from build123d import *

# Parameters (mm, degrees)
F1_DEPTH = 12.7
F2_DEPTH = 12.7
F4_DEPTH = 25.4
F6_DEPTH = 25.4
F8_DEPTH = 25.4


with BuildPart() as f1:
    # F0 (on Right) → F1 (new body)
    with BuildSketch(Plane.YZ):
        Polygon((304.799962, -64.221394), (304.799962, 304.800038), (266.7, 304.85419), (-42.510699, -10.741028), (-60.690689, -14.973944), (-60.690689, -19.789347), (-60.690689, -29.296394), (-60.690689, -64.221394), align=None)
        Polygon((-86.090689, -64.221394), (-60.690689, -64.221394), (-60.690689, -29.296394), (-60.690689, -19.789347), (-60.690689, -14.973944), (-86.090689, -14.973944), align=None)
    extrude(amount=F1_DEPTH)

    # F0 (on Right) → F2 (join)
    with BuildSketch(Plane.YZ):
        Polygon((304.799962, -64.221394), (304.799962, 304.800038), (266.7, 304.85419), (-42.510699, -10.741028), (-60.690689, -14.973944), (-60.690689, -19.789347), (-60.690689, -29.296394), (-60.690689, -64.221394), align=None)
        Polygon((-86.090689, -64.221394), (-60.690689, -64.221394), (-60.690689, -29.296394), (-60.690689, -19.789347), (-60.690689, -14.973944), (-86.090689, -14.973944), align=None)
    extrude(amount=F2_DEPTH)

    # F3 (on face) → F4 (cut)
    with BuildSketch(Plane.YZ.offset(12.7)):
        with BuildLine():
            Line((260.440068, 273.135901), (272.189458, 261.271445))
            ThreePointArc((272.189458, 261.271445), (279.866661, 265.037294), (282.611404, 273.135901))
            Line((282.611404, 273.135901), (282.614132, 279.79518))
            ThreePointArc((282.614132, 279.79518), (285.773725, 284.060884), (280.770869, 285.835901))
            Line((280.770869, 285.835901), (276.240647, 285.835901))
            ThreePointArc((276.240647, 285.835901), (276.167259, 285.912573), (276.174208, 286.018478))
            ThreePointArc((276.174208, 286.018478), (275.105821, 290.411047), (270.654796, 289.620796))
            Line((270.654796, 289.620796), (267.401841, 288.920168))
            ThreePointArc((267.401841, 288.920168), (266.952991, 289.962034), (266.735415, 291.075412))
            Line((266.735415, 291.075412), (266.735415, 304.926464))
            Line((266.735415, 304.926464), (243.648279, 281.326502))
            Line((243.648279, 281.326502), (252.004404, 281.326502))
            ThreePointArc((252.004404, 281.326502), (253.441245, 280.731343), (254.036404, 279.294502))
            Line((254.036404, 279.294502), (254.036404, 273.135901))
            Line((254.036404, 273.135901), (260.440068, 273.135901))
        make_face()
        with BuildLine():
            Line((177.841234, 200.373568), (177.841234, 214.224619))
            Line((177.841234, 214.224619), (154.754098, 190.624658))
            Line((154.754098, 190.624658), (163.110223, 190.624658))
            ThreePointArc((163.110223, 190.624658), (164.547063, 190.029499), (165.142223, 188.592658))
            Line((165.142223, 188.592658), (165.142223, 182.434057))
            Line((165.142223, 182.434057), (171.545887, 182.434057))
            Line((171.545887, 182.434057), (183.295277, 170.569601))
            ThreePointArc((183.295277, 170.569601), (190.972479, 174.33545), (193.717223, 182.434057))
            Line((193.717223, 182.434057), (193.719951, 189.093336))
            ThreePointArc((193.719951, 189.093336), (196.879544, 193.35904), (191.876687, 195.134057))
            Line((191.876687, 195.134057), (187.346465, 195.134057))
            ThreePointArc((187.346465, 195.134057), (187.273078, 195.210729), (187.280027, 195.316634))
            ThreePointArc((187.280027, 195.316634), (186.211639, 199.709203), (181.760615, 198.918952))
            Line((181.760615, 198.918952), (178.507659, 198.218324))
            ThreePointArc((178.507659, 198.218324), (178.05881, 199.26019), (177.841234, 200.373568))
        make_face()
        with BuildLine():
            Line((88.947052, 109.671724), (88.947052, 123.522775))
            Line((88.947052, 123.522775), (65.859917, 99.922814))
            Line((65.859917, 99.922814), (74.216041, 99.922814))
            ThreePointArc((74.216041, 99.922814), (75.652882, 99.327655), (76.248041, 97.890814))
            Line((76.248041, 97.890814), (76.248041, 91.732213))
            Line((76.248041, 91.732213), (82.651706, 91.732213))
            Line((82.651706, 91.732213), (94.401095, 79.867757))
            ThreePointArc((94.401095, 79.867757), (102.078298, 83.633606), (104.823041, 91.732213))
            Line((104.823041, 91.732213), (104.82577, 98.391492))
            ThreePointArc((104.82577, 98.391492), (107.985362, 102.657196), (102.982506, 104.432213))
            Line((102.982506, 104.432213), (98.452284, 104.432213))
            ThreePointArc((98.452284, 104.432213), (98.378896, 104.508885), (98.385845, 104.61479))
            ThreePointArc((98.385845, 104.61479), (97.317458, 109.007359), (92.866434, 108.217108))
            Line((92.866434, 108.217108), (89.613478, 107.51648))
            ThreePointArc((89.613478, 107.51648), (89.164628, 108.558346), (88.947052, 109.671724))
        make_face()
        with BuildLine():
            Line((0.052871, 18.96988), (0.052871, 32.820931))
            Line((0.052871, 32.820931), (-23.034265, 9.22097))
            Line((-23.034265, 9.22097), (-14.67814, 9.22097))
            ThreePointArc((-14.67814, 9.22097), (-13.241299, 8.625811), (-12.64614, 7.18897))
            Line((-12.64614, 7.18897), (-12.64614, 1.030369))
            Line((-12.64614, 1.030369), (-6.242476, 1.030369))
            Line((-6.242476, 1.030369), (5.506914, -10.834087))
            ThreePointArc((5.506914, -10.834087), (13.184117, -7.068238), (15.92886, 1.030369))
            Line((15.92886, 1.030369), (15.931588, 7.689648))
            ThreePointArc((15.931588, 7.689648), (19.091181, 11.955352), (14.088325, 13.730369))
            Line((14.088325, 13.730369), (9.558103, 13.730369))
            ThreePointArc((9.558103, 13.730369), (9.484715, 13.80704), (9.491664, 13.912946))
            ThreePointArc((9.491664, 13.912946), (8.423277, 18.305515), (3.972252, 17.515264))
            Line((3.972252, 17.515264), (0.719297, 16.814636))
            ThreePointArc((0.719297, 16.814636), (0.270447, 17.856502), (0.052871, 18.96988))
        make_face()
    extrude(amount=-F4_DEPTH, mode=Mode.SUBTRACT)

    # F5 (on face) → F6 (cut)
    with BuildSketch(Plane.YZ.offset(12.7)):
        with BuildLine():
            Line((292.099962, -26.121394), (304.799962, -26.121394))
            Line((304.799962, -26.121394), (304.799962, 11.978606))
            Line((304.799962, 11.978606), (292.099962, 11.978606))
            ThreePointArc((292.099962, 11.978606), (288.905703, 9.513217), (290.481334, 5.798542))
            ThreePointArc((290.481334, 5.798542), (291.665592, 4.634162), (292.099962, 3.031173))
            Line((292.099962, 3.031173), (292.099962, -17.173962))
            ThreePointArc((292.099962, -17.173962), (291.665592, -18.77695), (290.481334, -19.941331))
            ThreePointArc((290.481334, -19.941331), (288.905703, -23.656006), (292.099962, -26.121394))
        make_face()
        with BuildLine():
            Line((304.799962, 94.528606), (292.099962, 94.528606))
            ThreePointArc((292.099962, 94.528606), (288.905703, 92.063217), (290.481334, 88.348542))
            ThreePointArc((290.481334, 88.348542), (291.665592, 87.184162), (292.099962, 85.581173))
            Line((292.099962, 85.581173), (292.099962, 65.376038))
            ThreePointArc((292.099962, 65.376038), (291.665592, 63.77305), (290.481334, 62.608669))
            ThreePointArc((290.481334, 62.608669), (288.905703, 58.893994), (292.099962, 56.428606))
            Line((292.099962, 56.428606), (304.799962, 56.428606))
            Line((304.799962, 56.428606), (304.799962, 94.528606))
        make_face()
        with BuildLine():
            Line((304.799962, 177.078606), (292.099962, 177.078606))
            ThreePointArc((292.099962, 177.078606), (288.905703, 174.613217), (290.481334, 170.898542))
            ThreePointArc((290.481334, 170.898542), (291.665592, 169.734162), (292.099962, 168.131173))
            Line((292.099962, 168.131173), (292.099962, 147.926038))
            ThreePointArc((292.099962, 147.926038), (291.665592, 146.32305), (290.481334, 145.158669))
            ThreePointArc((290.481334, 145.158669), (288.905703, 141.443994), (292.099962, 138.978606))
            Line((292.099962, 138.978606), (304.799962, 138.978606))
            Line((304.799962, 138.978606), (304.799962, 177.078606))
        make_face()
        with BuildLine():
            Line((304.799962, 259.628606), (292.099962, 259.628606))
            ThreePointArc((292.099962, 259.628606), (288.905703, 257.163217), (290.481334, 253.448542))
            ThreePointArc((290.481334, 253.448542), (291.665592, 252.284162), (292.099962, 250.681173))
            Line((292.099962, 250.681173), (292.099962, 230.476038))
            ThreePointArc((292.099962, 230.476038), (291.665592, 228.87305), (290.481334, 227.708669))
            ThreePointArc((290.481334, 227.708669), (288.905703, 223.993994), (292.099962, 221.528606))
            Line((292.099962, 221.528606), (304.799962, 221.528606))
            Line((304.799962, 221.528606), (304.799962, 259.628606))
        make_face()
    extrude(amount=-F6_DEPTH, mode=Mode.SUBTRACT)

    # F7 (on face) → F8 (cut)
    with BuildSketch(Plane.YZ.offset(12.7)):
        with BuildLine():
            Line((-78.322477, -29.296394), (-86.090689, -29.296394))
            Line((-86.090689, -29.296394), (-86.090689, -51.521394))
            Line((-86.090689, -51.521394), (-78.322477, -51.521394))
            ThreePointArc((-78.322477, -51.521394), (-77.191976, -51.864906), (-76.4437, -52.779299))
            ThreePointArc((-76.4437, -52.779299), (-71.055822, -53.856261), (-72.132784, -48.468383))
            ThreePointArc((-72.132784, -48.468383), (-73.047177, -47.720107), (-73.390689, -46.589606))
            Line((-73.390689, -46.589606), (-73.390689, -34.228182))
            ThreePointArc((-73.390689, -34.228182), (-73.047177, -33.097682), (-72.132784, -32.349406))
            ThreePointArc((-72.132784, -32.349406), (-71.055822, -26.961528), (-76.4437, -28.03849))
            ThreePointArc((-76.4437, -28.03849), (-77.191976, -28.952883), (-78.322477, -29.296394))
        make_face()
    extrude(amount=-F8_DEPTH, mode=Mode.SUBTRACT)


solid = f1.part
Geometry check sheet. Reference: the model listing, model coordinates, mm. A direction names the side the tool comes from. Round coordinates to 2 decimals unless told otherwise and drop trailing zeros. Loops run counter-clockwise (first coordinate to the right, second up) from the corner with the lowest first, then second, coordinate; pieces in that order, holes last.
Item 1: Thickness scan on line 1 (Z direction, x = 5, y = 81.5); line 2 (Y direction, x = 10.5, z = 95); line 3 (Y direction, x = 11.5, z = 265). Record the ranges inside material, lowest first.
Item 2: Gauge pin test, flat ends, axial feed: pin 1 (1.5 mm diameter, centred on x = 9.5, z = 92.5, fed in from +Y); pin 2 (6 mm diameter, centred on x = 6.5, y = 130, fed in from +Z); pin 3 (1.9 mm diameter, centred on x = 7, y = 257.5, fed in from +Z). Record the tip position at first contact, or that the pin passes through.
Item 3: Cross-section at B-B on y = 131. Record the boundary of the cut face in (x, z).
Item 4: Access from +Z, -Z, +X, -X, +Y, -Y to the whole of each face (thin tool, end or side, straight path). Record for faces 4 (the flat face through (6, 292.1, -7)), 5 (the flat face through (6, 266.735, 298)), 6 (the flat face through (6, -73.391, -40)), 7 (the flat face through (6.44, 266.23, 267.29)).
Item 5: Mould release check, pull along Z, two halves, no side actions. Record for faces 1 (the cylindrical face through (6.44, 190.89, 174.24)), 2 (the flat face through (6, 0.053, 26)), 3 (the flat face through (6.261, 211.205, 248.214)): pulls with the +Z half, pulls with the -Z half, needs draft (parallel to the pull), parting line crosses it, or undercut.
Item 6: Cross-section at A-A on z = 114.5. Record the boundary of the cut face in (x, y), then the cut area to 3 significant figures.
Answer sheet:
1. line 1: z = -64.22 to 91.73
1. line 2: y = 61.09 to 76.25, 104.82 to 304.8
1. line 3: y = 227.65 to 268.5, 279.83 to 304.8
2. pin 1: stops at y = 289.49
2. pin 2: stops at z = 168.39
2. pin 3: stops at z = 273.14
3. outline: (0, -64.22) - (12.7, -64.22) - (12.7, 166.35) - (0, 166.35) - close
4. face 4: +X, -X, +Y
4. face 5: +Z, +X, -X, -Y
4. face 6: +X, -X, -Y
4. face 7: +X, -X
5. face 1: undercut
5. face 2: needs draft
5. face 3: pulls with the +Z half
6. outline: (0, 88.95) - (12.7, 88.95) - (12.7, 304.8) - (0, 304.8) - close
6. area: 2,740 mm2
